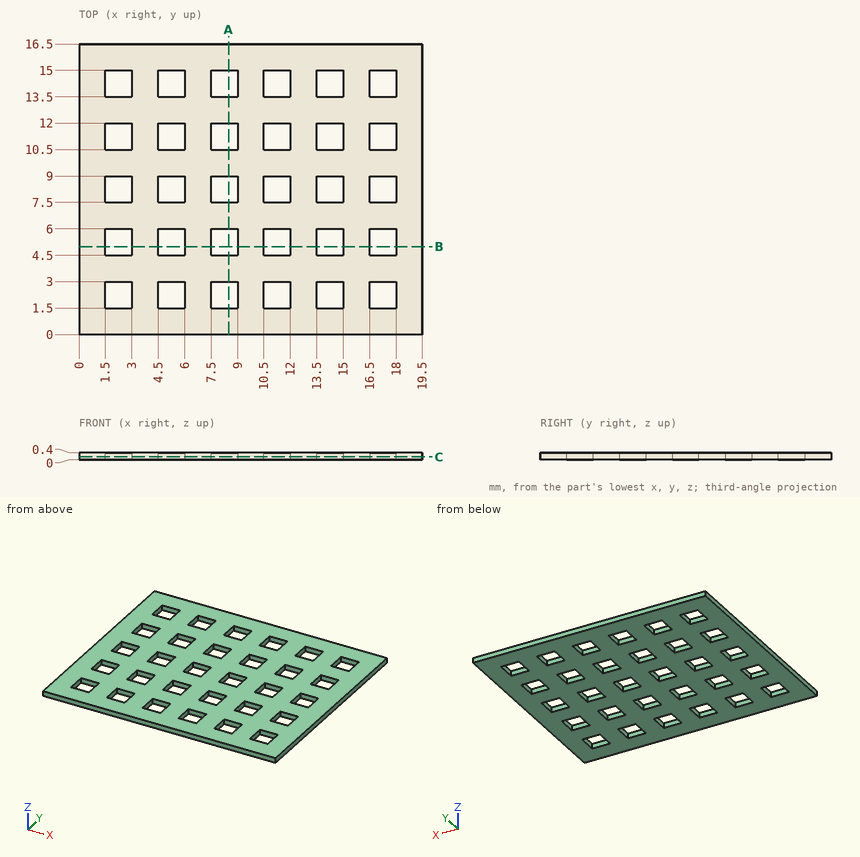
Can you work these out from the drawing? Everything is in mm from the part's minimum corner. Coordinates: 2 decimals unless noted, no trailing zeros. Write each loop counter-clockwise with the first axis right and the second up, starting at its lowest first coordinate (ties: lowest second). Pieces come first, ordered by that corner, then holes. Notation, with made-up numbers: (-30, 85.25) - (22, 85.25) arc R16 ccw to (22, 104.25) - close; hole circle Ø4 at (19, 54.5). An arc over 180 degrees is marked (long way). One line per item, written item: value.
1) Suppose I cut it at A-A on x = 8.5. Write out the boundary of the cut face in (y, z).
Model answer:
outline: (0, 0) - (1.5, 0) - (1.5, 0.4) - (0, 0.4) - close; (3, 0) - (4.5, 0) - (4.5, 0.4) - (3, 0.4) - close; (6, 0) - (7.5, 0) - (7.5, 0.4) - (6, 0.4) - close; (9, 0) - (10.5, 0) - (10.5, 0.4) - (9, 0.4) - close; (12, 0) - (13.5, 0) - (13.5, 0.4) - (12, 0.4) - close; (15, 0) - (16.5, 0) - (16.5, 0.4) - (15, 0.4) - close
2) Suppose I cut it at B-B on y = 5. Write out the boundary of the cut face in (x, z), and give its area (3 significant figures).
Model answer:
outline: (0, 0) - (1.5, 0) - (1.5, 0.4) - (0, 0.4) - close; (3, 0) - (4.5, 0) - (4.5, 0.4) - (3, 0.4) - close; (6, 0) - (7.5, 0) - (7.5, 0.4) - (6, 0.4) - close; (9, 0) - (10.5, 0) - (10.5, 0.4) - (9, 0.4) - close; (12, 0) - (13.5, 0) - (13.5, 0.4) - (12, 0.4) - close; (15, 0) - (16.5, 0) - (16.5, 0.4) - (15, 0.4) - close; (18, 0) - (19.5, 0) - (19.5, 0.4) - (18, 0.4) - close
area: 4.20 mm²
3) I need wall thicknesses on line 1 along Y through (x, z) = (14, 0.3). Which ranges of the line are inside material? Lowest first, please.
Model answer:
line 1: y = 0 to 1.5, 3 to 4.5, 6 to 7.5, 9 to 10.5, 12 to 13.5, 15 to 16.5
4) Suppose I cut it at C-C on z = 0.15. State how many separate pieces and enclosed holes the cut face has, and give its area (3 significant figures).
Model answer:
separate pieces: 1
enclosed holes: 30
area: 254 mm²
